from build123d import *

# Parameters (mm, degrees)
SKETCH1_R           = 50.2
SKETCH1_R_2         = 44.15
BOSS_EXTRUDE1_DEPTH = 1.6
SKETCH2_R           = 1.8
SKETCH2_R_2         = 1.2
CUT_EXTRUDE1_DEPTH  = 2.6
CIRPATTERN1_COUNT   = 4


with BuildPart() as part:
    # Sketch1 → Boss-Extrude1 (new body)
    with BuildSketch(Plane.XY):
        Circle(SKETCH1_R)
        Circle(SKETCH1_R_2, mode=Mode.SUBTRACT)
    extrude(amount=BOSS_EXTRUDE1_DEPTH)

    # Sketch2 → Cut-Extrude1 (cut, through all)
    with BuildSketch(Plane.XY.offset(1.6)):
        with Locations((-45.963155758, 9.769770352)):
            Circle(SKETCH2_R)
        with Locations((-9.769770352, 45.963155758)):
            Circle(SKETCH2_R)
        with Locations((-42.333815877, 20.393825862)):
            Circle(SKETCH2_R_2)
        with Locations((-43.914877634, 16.719558081)):
            Circle(SKETCH2_R_2)
        with Locations((-20.393825862, 42.333815877)):
            Circle(SKETCH2_R_2)
        with Locations((-16.719558081, 43.914877634)):
            Circle(SKETCH2_R_2)
        with Locations((-46.99, 0)):
            Circle(SKETCH2_R)
        with Locations((0, 46.99)):
            Circle(SKETCH2_R)
    cut_extrude1 = extrude(amount=-CUT_EXTRUDE1_DEPTH, mode=Mode.SUBTRACT)

    # CirPattern1: Cut-Extrude1 ×4 about axis
    cirpattern1_axis = Axis((0, 0, 0), (0, 0, 1))
    for i in range(1, CIRPATTERN1_COUNT):
        add(cut_extrude1.rotate(cirpattern1_axis, i * 360 / CIRPATTERN1_COUNT), mode=Mode.SUBTRACT)


solid = part.part
Read the model definition and answer for the solid it produces. Units are mm, in the model's axes. Round coordinates to 2 decimals unless told otherwise and drop trailing zeros. Write each loop counter-clockwise with the first axis right and the second up, starting at its lowest first coordinate (ties: lowest second). Pieces come first, ordered by that corner, then holes. Notation, with made-up numbers: (63, 40.25) - (115, 40.25) arc R6 ccw to (115, 48.25) - close; hole circle Ø3 at (-35.75, 75). An arc over 180 degrees is marked (long way). One line per question, with ' | ' between items. Start each with the question number.
1. Section A-A (y = 0) is taken. Determine the outline of the cut face in (x, z).
2. Section D-D (y = -23.5) is taken. Determine the outline of the cut face in (x, z), and give its area (3 significant figures).
3. Section C-C (z = 0.7) is taken. Give the number of separate pieces and of enclosed holes in the cut face, and give its area (3 significant figures).
4. For a pull along X with two mould halves and no side action, classify faces 1 (the face through (33, -30, 0)), 2 (the face through (46.37, -19.23, 0.79)), 3 (the face through (-47.39, 8.67, 0.81)) as +X half, -X half, draft (parallel to the pull), parting line (faces both ways), or undercut.
5. Find the intervals of material crossed by probe 1 along Y at (x, z) = (0, 0.5); probe 2 along Y at (x, z) = (1.5, 0.2); probe 3 along X at (y, z) = (17.5, 0.5), in increasing order. Write a range as [from, to].
6. Section B-B (x = -30) is taken. Determine the outline of the cut face in (y, z).
Filled in:
1) outline: (-50.2, 0) - (-48.79, 0) - (-48.79, 1.6) - (-50.2, 1.6) - close; (-45.19, 0) - (-44.15, 0) - (-44.15, 1.6) - (-45.19, 1.6) - close; (44.15, 0) - (45.19, 0) - (45.19, 1.6) - (44.15, 1.6) - close; (48.79, 0) - (50.2, 0) - (50.2, 1.6) - (48.79, 1.6) - close
2) outline: (-44.36, 0) - (-37.38, 0) - (-37.38, 1.6) - (-44.36, 1.6) - close; (37.38, 0) - (44.36, 0) - (44.36, 1.6) - (37.38, 1.6) - close | area: 22.3 mm²
3) separate pieces: 1 | enclosed holes: 29 | area: 1,600 mm²
4) face 1: draft | face 2: parting line | face 3: undercut
5) probe 1: [-50.2, -48.79], [-45.19, -44.15], [44.15, 45.19], [48.79, 50.2] | probe 2: [-50.18, -47.98], [-46, -44.12], [44.12, 46], [47.98, 50.18] | probe 3: [-47.05, -44.83], [-43, -40.53], [40.53, 43], [44.83, 47.05]
6) outline: (-40.25, 0) - (-32.39, 0) - (-32.39, 1.6) - (-40.25, 1.6) - close; (32.39, 0) - (40.25, 0) - (40.25, 1.6) - (32.39, 1.6) - close
